from build123d import *

# Parameters (mm, degrees)
SKETCH_4_R               = 5.5
SKETCH_4_R_2             = 1.5
EXTRUDE_1_DEPTH          = 2.93
EXTRUDE_START            = 2
SKETCH_5_R               = 2.5
SKETCH_5_R_2             = 1.5
EXTRUDE_2_DEPTH          = 2
SKETCH_6_R               = 4.3
CUT_EXTRUDE_1_DEPTH      = 1.7
SKETCH_7_W               = 1.2
SKETCH_7_H               = 1.242066229
CUT_EXTRUDE_2_DEPTH      = 1.33
PATTERN_CIRCULAR_1_COUNT = 20


with BuildPart() as part:
    # 草图4 → 凸台-拉伸1 (new body)
    with BuildSketch(Plane(origin=(0, 0, 0), x_dir=(1, 0, 0), z_dir=(0, 1, 0))):
        with Locations(Location((0, 0, 0), (0, 0, 90))):
            Circle(SKETCH_4_R)
        with Locations(Location((0, 0, 0), (0, 0, 90))):
            Circle(SKETCH_4_R_2, mode=Mode.SUBTRACT)
    extrude(amount=EXTRUDE_1_DEPTH)

    # 草图5 → 凸台-拉伸2 (add)
    with BuildSketch(Plane.XZ.offset(EXTRUDE_START)):
        with Locations(Location((0, 0, 0), (0, 0, 90))):
            Circle(SKETCH_5_R)
        with Locations(Location((0, 0, 0), (0, 0, 270))):
            Circle(SKETCH_5_R_2, mode=Mode.SUBTRACT)
    extrude(amount=-EXTRUDE_2_DEPTH)

    # 草图6 → 切除-拉伸1 (cut)
    with BuildSketch(Plane(origin=(0, 2.93, 0), x_dir=(1, 0, 0), z_dir=(0, 1, 0))):
        with Locations(Location((0, 0, 0), (0, 0, 270))):
            Circle(SKETCH_6_R)
    extrude(amount=-CUT_EXTRUDE_1_DEPTH, mode=Mode.SUBTRACT)

    # 草图7 → 切除-拉伸2 (cut)
    with BuildSketch(Plane(origin=(0, 2.93, 0), x_dir=(1, 0, 0), z_dir=(0, 1, 0))):
        with Locations((0, 4.878966886)):
            Rectangle(SKETCH_7_W, SKETCH_7_H)
    cut_extrude_2 = extrude(amount=-CUT_EXTRUDE_2_DEPTH, mode=Mode.SUBTRACT)

    # 阵列(圆周)1: 切除-拉伸2 ×20 about axis
    pattern_circular_1_axis = Axis((0, 0, 0), (0, 1, 0))
    for i in range(1, PATTERN_CIRCULAR_1_COUNT):
        add(cut_extrude_2.rotate(pattern_circular_1_axis, i * 360 / PATTERN_CIRCULAR_1_COUNT), mode=Mode.SUBTRACT)


solid = part.part
Input: part model. Units: mm. Frame: model coordinates. A direction names the side the tool comes from. Give positions to 0.01 mm unless a question says otherwise; leave off trailing zeros. Order: outer loops, then holes, each group sorted by start corner. A loop starts at its lowest first (then second) coordinate and runs counter-clockwise, first axis right, second up. Notation, with made-up numbers: (65, 18) - (121, 18) arc R19 cw to (121, 32) - close; hole circle Ø8 at (41, 88.25). An arc over 180 degrees is marked (long way). Answer as a JSON object with one key per item and string values. Group by question number.
Q1. Cut plane B-B, the plane z = 0. Output: boundary loops of the cut face in (x, y).
Q2. Mould query, pull axis X, two halves, no side actions, for faces 1 (the face through (4.5, 2.93, -2.3)), 2 (the face through (4.43, 2.27, 2.07)), 3 (the face through (-4.7, 1.6, -1.5)). Classes: pulls with the +X half, pulls with the -X half, needs draft (parallel to the pull), parting line crosses it, or undercut.
Q3. First-contact query: pin 1 Ø2 at (x, z) = (-0.5, -0.5) entering from +Y; pin 2 Ø2 at (y, z) = (-0.5, -3) entering from -X; pin 3 Ø2 at (y, z) = (-0.5, -4) entering from -X. Flat tips, straight axial feed; report the tip coordinate or a pass-through.
Q4. Cut plane A-A, the plane x = 0. Output: boundary loops of the cut face in (y, z).
Q5. Cut plane D-D, the plane y = 2.55. Count the separate pieces of the cut face and the enclosed holes in it, then the cut area to 3 significant figures.
Q6. Set-up query: faces 4 (the face through (-4.43, 2.27, -2.07)), 5 (the face through (-5, 1.6, 0)), 6 (the face through (-2.07, 2.27, 4.43)), 7 (the face through (0.93, 2.27, 4.8)). Return all of +Z, -Z, +X, -X, +Y, -Y with unobstructed straight access to the full face (end or side cutting, diameter ignored); none if empty.
Q7. Line query: probe 1 along X at (y, z) = (0.05, 0); probe 2 along Y at (x, z) = (2.25, -0.5); probe 3 along Y at (x, z) = (-0.5, -4.5). Output: solid intervals per line, ascending.
Q8. Cut plane C-C, the plane y = -0.8. Output: boundary loops of the cut face in (x, z).
Results:
{
 "1": {"outline": "(-5.5, 0) - (-2.5, 0) - (-2.5, -2) - (-1.5, -2) - (-1.5, 1.23) - (-4.3, 1.23) - (-4.3, 1.6) - (-5.5, 1.6) - close; (1.5, -2) - (2.5, -2) - (2.5, 0) - (5.5, 0) - (5.5, 1.6) - (4.3, 1.6) - (4.3, 1.23) - (1.5, 1.23) - close"},
 "2": {"face 1": "needs draft", "face 2": "pulls with the +X half", "face 3": "undercut"},
 "3": {"pin 1": "y = 1.23", "pin 2": "x = -5.07", "pin 3": "x = -4.52"},
 "4": {"outline": "(-2, -2.5) - (0, -2.5) - (0, -5.5) - (1.6, -5.5) - (1.6, -4.3) - (1.23, -4.3) - (1.23, -1.5) - (-2, -1.5) - close; (-2, 1.5) - (1.23, 1.5) - (1.23, 4.3) - (1.6, 4.3) - (1.6, 5.5) - (0, 5.5) - (0, 2.5) - (-2, 2.5) - close"},
 "5": {"separate pieces": "20", "enclosed holes": "0", "area": "8.07 mm^2"},
 "6": {"face 4": "-X, +Y", "face 5": "+X, -X, +Y", "face 6": "+Z, +Y", "face 7": "+Y"},
 "7": {"probe 1": "-5.5 to -1.5, 1.5 to 5.5", "probe 2": "-2 to 1.23", "probe 3": "0 to 1.6"},
 "8": {"outline": "circle Ø5 at (0, 0); hole circle Ø3 at (0, 0)"}
}
